Here's how the part is built. I have some questions about the finished solid (model axes, mm). Face numbers are marked on the shaded views. Round coordinates to 2 decimals unless told otherwise and drop trailing zeros. Loops run counter-clockwise (first coordinate to the right, second up) from the corner with the lowest first, then second, coordinate; pieces in that order, holes last. Notation, with made-up numbers: (45, 21.5) -> (75, 21.5) arc R33 ccw to (75, 49.5) -> close; hole circle Ø11 at (4.25, 48). An arc over 180 degrees is marked (long way). One line per item, written item: value. Start each with the question number.
```python
from build123d import *

# Parameters (mm, degrees)
SKETCH_1_R          = 1.5
EXTRUDE_1_DEPTH     = 30
SKETCH_1_2_R        = 1.5
EXTRUDE_2_DEPTH     = 36
SKETCH_2_R          = 1.5
CUT_EXTRUDE_1_DEPTH = 8


with BuildPart() as part:
    # Sketch 1 → Extrude 1 (new body)
    with BuildSketch(Plane(origin=(0, 0, 0), x_dir=(1, 0, 0), z_dir=(0, 1, 0))):
        Polygon((1.248465648, 2.278449808), (-1.348962591, 2.220427871), (-2.597428239, -0.058021937), (-1.248465648, -2.278449808), (1.348962591, -2.220427871), (2.597428239, 0.058021937), align=None)
        with Locations(Location((0, 0, 0), (0, 0, 270))):
            Circle(SKETCH_1_R, mode=Mode.SUBTRACT)
    extrude(amount=EXTRUDE_1_DEPTH)

    # Sketch 1_2 → Extrude 2 (add)
    with BuildSketch(Plane(origin=(0, 0, 0), x_dir=(1, 0, 0), z_dir=(0, 1, 0))):
        with Locations(Location((0, 0, 0), (0, 0, 270))):
            Circle(SKETCH_1_2_R)
    extrude(amount=EXTRUDE_2_DEPTH)

    # Sketch 2 → Cut-Extrude 1 (cut)
    with BuildSketch(Plane.XZ):
        with Locations(Location((0, 0, 0), (0, 0, 90))):
            Circle(SKETCH_2_R)
    extrude(amount=-CUT_EXTRUDE_1_DEPTH, mode=Mode.SUBTRACT)


solid = part.part
```
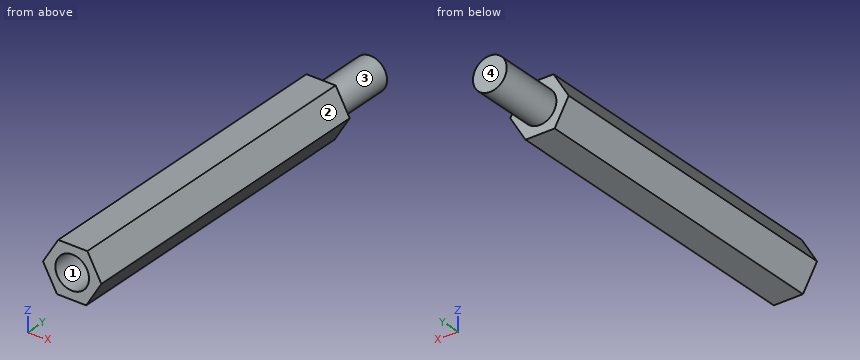
Q1. If we mould it in two halves opening along X, with no side actions, what happens to the marked faces 1, 2, 3 and 4? For each: released by +X, released by -X, zero draft, split by the parting line, or undercut.
Q2. If I drill on line 1 along Y through (x, z) = (-1.7, 0.4); line 2 along Z through (x, y) = (0.8, 2); line 3 along Y through (x, z) = (0.2, -1), over which ranges is the centre line in solid material (lowest first)?
Q3. I want a section at C-C on z = -0.8. Please give me the cut outline in (x, y).
Q4. Will this pin go through, and if not, where does the flat tip stop? P1, Ø1.5, axis at x = -1.5, y = 7.5, coming from the -Z side.
Q5. I want a section at A-A on x = 0. Please give me the cut outline in (y, z), plus the area to 3 significant figures.
Q6. I want a section at D-D on z = 1.8. Please give me the cut outline in (x, y).
Q7. I want a section at B-B on y = 24. Please give me the cut outline in (x, z).
Answers below:
1. face 1: undercut
1. face 2: released by +X
1. face 3: split by the parting line
1. face 4: zero draft
2. line 1: y = 0 to 30
2. line 2: z = -2.27 to -1.27, 1.27 to 2.23
2. line 3: y = 8 to 36
3. outline: (-2.13, 0) -> (-1.27, 0) -> (-1.27, 8) -> (1.27, 8) -> (1.27, 0) -> (2.15, 0) -> (2.15, 30) -> (1.27, 30) -> (1.27, 36) -> (-1.27, 36) -> (-1.27, 30) -> (-2.13, 30) -> close
4. P1: stops at z = -2.23
5. outline: (0, -2.25) -> (30, -2.25) -> (30, -1.5) -> (36, -1.5) -> (36, 1.5) -> (30, 1.5) -> (30, 2.25) -> (0, 2.25) -> (0, 1.5) -> (8, 1.5) -> (8, -1.5) -> (0, -1.5) -> close
5. area: 129 mm^2
6. outline: (-1.54, 0) -> (1.58, 0) -> (1.58, 30) -> (-1.54, 30) -> close
7. outline: (-2.6, 0.06) -> (-1.35, -2.22) -> (1.25, -2.28) -> (2.6, -0.06) -> (1.35, 2.22) -> (-1.25, 2.28) -> close
